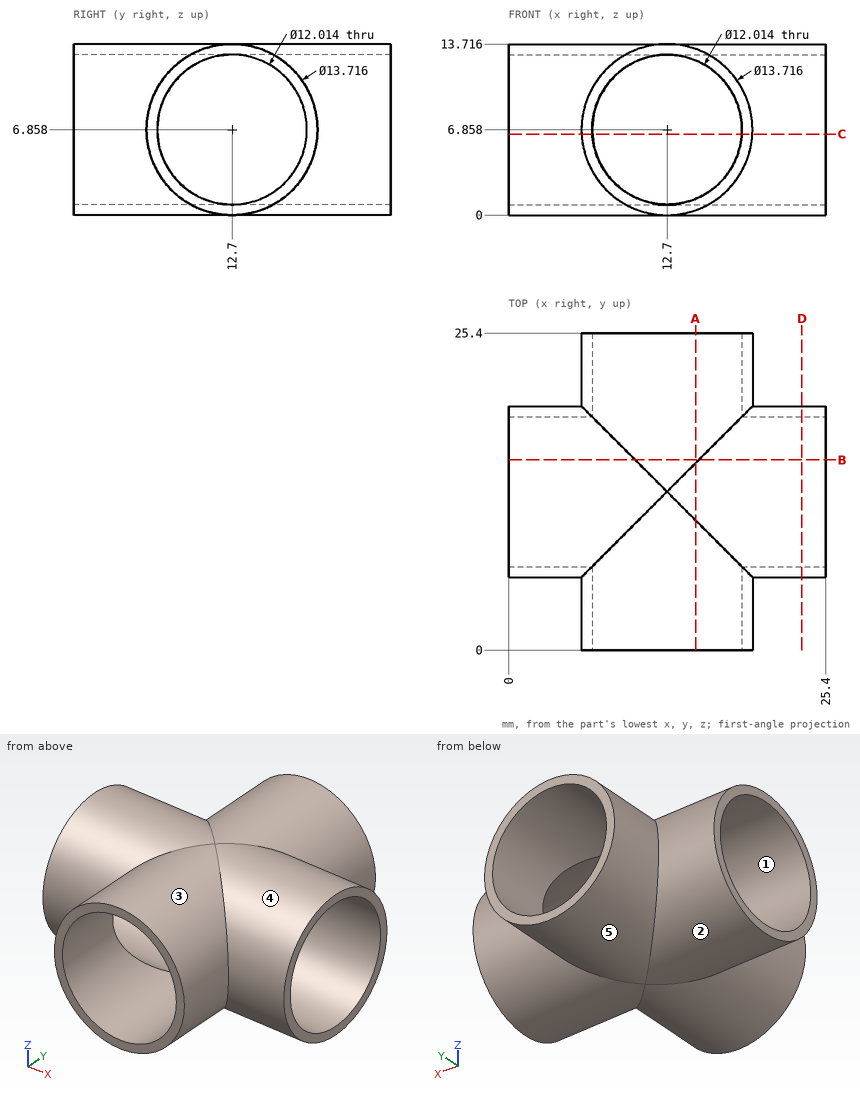
Answer from the drawing. Dimensions are ordinates in mm from the lowest x, y and z of the part. A direction names the side the tool comes from. Coordinates: 2 decimals unless noted, no trailing zeros. Loops run counter-clockwise (first coordinate to the right, second up) from the corner with the lowest first, then second, coordinate; pieces in that order, holes last.
1) Section C-C (z = 6.5) is taken. Give the vertices of the cut face in (x, y), plus the area to 3 significant figures.
Results:
outline: (0, 5.85) - (5.85, 5.85) - (5.85, 0) - (6.7, 0) - (6.7, 6.7) - (0, 6.7) - close; (0, 18.7) - (6.7, 18.7) - (6.7, 25.4) - (5.85, 25.4) - (5.85, 19.55) - (0, 19.55) - close; (18.7, 0) - (19.55, 0) - (19.55, 5.85) - (25.4, 5.85) - (25.4, 6.7) - (18.7, 6.7) - close; (18.7, 18.7) - (25.4, 18.7) - (25.4, 19.55) - (19.55, 19.55) - (19.55, 25.4) - (18.7, 25.4) - close
area: 42.8 mm2
2) Section D-D (x = 23.5) is taken. Give the vertices of the cut face in (y, z).
Results:
outline: circle Ø13.72 at (12.7, 6.86); hole circle Ø12.01 at (12.7, 6.86)
3) For a pull along Y with two mould halves and no side action, classify the marked faces 1 and 2 as +Y half, -Y half, draft (parallel to the pull), parting line (faces both ways), or undercut.
Results:
face 1: undercut
face 2: parting line
4) Flat-ended cylindrical pins translate along their axes: pin 1 (5 mm diameter, centred on x = 7.5, y = 19.5, fed in from -Z); pin 2 (10 mm diameter, centred on x = 4, y = 4, fed in from -Z); pin 3 (3 mm diameter, centred on y = 21.5, z = 5.5, fed in from +X). Find the tip coordinate at first contact, or state that the pin passes through.
Results:
pin 1: stops at z = 0.55
pin 2: stops at z = 1.08
pin 3: stops at x = 19.56
5) For the marked faces 3, 4 and 5, determine the directions among +Z, -Z, +X, -X, +Y, -Y from which every point of the face is accessible in a straight line to the end or side of a thin tool.
Results:
face 3: -Y
face 4: +X
face 5: +Y
6) Section B-B (y = 15.25) is taken. Give the vertices of the cut face in (x, z).
Results:
outline: (0, 0.49) - (10.15, 0.49) arc R6.86 ccw to (15.25, 0.49) - (25.4, 0.49) - (25.4, 1.42) - (15.25, 1.42) arc R6.01 cw to (10.15, 1.42) - (0, 1.42) - close; (0, 12.3) - (10.15, 12.3) arc R6.01 cw to (15.25, 12.3) - (25.4, 12.3) - (25.4, 13.22) - (15.25, 13.22) arc R6.86 ccw to (10.15, 13.22) - (0, 13.22) - close
7) Consider probe 1 along Z at (x, y) = (7.5, 12.7) (1 decimal); probe 2 along Y at (x, z) = (7.5, 10.25); probe 3 along Z at (x, y) = (14.25, 9.75). Determine where each line is inside the solid, lowest interval first.
Results:
probe 1: z = 0 to 0.9, 12.9 to 13.7
probe 2: y = 0 to 7.74, 17.66 to 25.4
probe 3: z = 0.18 to 1.05, 12.66 to 13.54
8) Section A-A (x = 15) is taken. Give the vertices of the cut face in (y, z).
Results:
outline: (0, 0.4) - (10.4, 0.4) arc R6.86 ccw to (15, 0.4) - (25.4, 0.4) - (25.4, 1.31) - (15, 1.31) arc R6.01 cw to (10.4, 1.31) - (0, 1.31) - close; (0, 12.41) - (10.4, 12.41) arc R6.01 cw to (15, 12.41) - (25.4, 12.41) - (25.4, 13.32) - (15, 13.32) arc R6.86 ccw to (10.4, 13.32) - (0, 13.32) - close
